Geometry: final body of the model. Coordinates: model frame, mm. Face numbers are marked on the shaded views. A direction names the side the tool comes from. Round coordinates to 2 decimals unless told otherwise and drop trailing zeros. Loops run counter-clockwise (first coordinate to the right, second up) from the corner with the lowest first, then second, coordinate; pieces in that order, holes last. Notation, with made-up numbers: (61, 22.25) - (111, 22.25) arc R32 ccw to (111, 50.25) - close; hole circle Ø3 at (19.25, -6). An arc over 180 degrees is marked (long way). Answer in a Markdown table with one row per item. Add a question column.
from build123d import *

# Parameters (mm, degrees)
SKETCH1_R           = 1.5
BOSS_EXTRUDE1_DEPTH = 1.6
SKETCH2_W           = 5
SKETCH2_H           = 25.4
BOSS_EXTRUDE2_DEPTH = 8


with BuildPart() as part:
    # Sketch1 → Boss-Extrude1 (new body)
    with BuildSketch(Plane(origin=(0, 0, 0), x_dir=(1, 0, 0), z_dir=(0, 1, 0))):
        with BuildLine():
            Line((1.5, 0), (98.5, 0))
            ThreePointArc((98.5, 0), (99.560660172, 0.439339828), (100, 1.5))
            Line((100, 1.5), (100, 78.5))
            ThreePointArc((100, 78.5), (99.560660172, 79.560660172), (98.5, 80))
            Line((98.5, 80), (1.5, 80))
            ThreePointArc((1.5, 80), (0.439339828, 79.560660172), (0, 78.5))
            Line((0, 78.5), (0, 1.5))
            ThreePointArc((0, 1.5), (0.439339828, 0.439339828), (1.5, 0))
        make_face()
        with Locations(Location((4, 4, 0), (0, 0, 270))):
            Circle(SKETCH1_R, mode=Mode.SUBTRACT)
        with Locations(Location((96, 76, 0), (0, 0, 270))):
            Circle(SKETCH1_R, mode=Mode.SUBTRACT)
        with Locations(Location((96, 4, 0), (0, 0, 270))):
            Circle(SKETCH1_R, mode=Mode.SUBTRACT)
        with Locations(Location((4, 76, 0), (0, 0, 270))):
            Circle(SKETCH1_R, mode=Mode.SUBTRACT)
    extrude(amount=BOSS_EXTRUDE1_DEPTH)

    # Sketch2 → Boss-Extrude2 (add)
    with BuildSketch(Plane(origin=(0, 1.6, 0), x_dir=(1, 0, 0), z_dir=(0, 1, 0))):
        with Locations((14.261833114, 15.332116758)):
            Rectangle(SKETCH2_W, SKETCH2_H)
        with Locations((13.597516255, 57.170048516)):
            Rectangle(SKETCH2_W, SKETCH2_H)
        with Locations((89.647028889, 60.563234223)):
            Rectangle(SKETCH2_W, SKETCH2_H)
        with Locations((86.389643886, 19.240978761)):
            Rectangle(SKETCH2_W, SKETCH2_H)
        with Locations((42.820913135, 59.911757222)):
            Rectangle(SKETCH2_W, SKETCH2_H)
        with Locations((68.613628586, 59.818689079)):
            Rectangle(SKETCH2_W, SKETCH2_H)
        with Locations((35.760574132, 15.239048615)):
            Rectangle(SKETCH2_W, SKETCH2_H)
        with Locations((64.518630297, 14.959844186)):
            Rectangle(SKETCH2_W, SKETCH2_H)
    extrude(amount=BOSS_EXTRUDE2_DEPTH)


solid = part.part
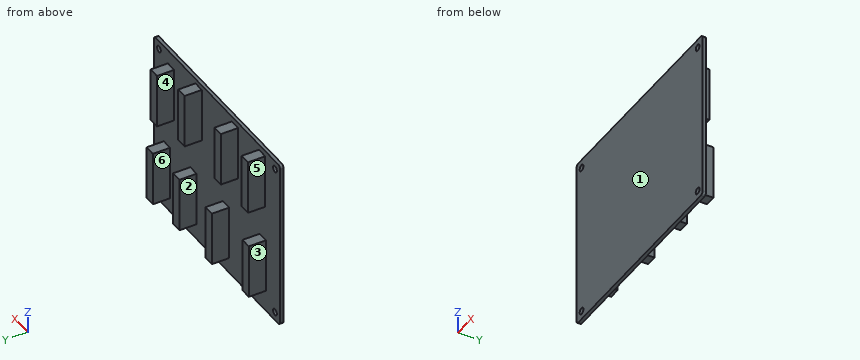
1) Material intervals for line 1 along X through (y, z) = (0.7, -4); line 2 along X through (y, z) = (5.25, -4); line 3 along Z through (x, y) = (96, 1.05), sorted ascending. Write a range as from..to.
2) Pull-direction query (X, two-part tool) for the marked faces 1, 2 and 3; classes: pulls with the +X half, pulls with the -X half, needs draft (parallel to the pull), parting line crosses it, or undercut.
3) Section D-D, the plane x = 14. Return the cut outline in (y, z).
4) Reachability of the marked faces 4, 5 and 6 from +Z, -Z, +X, -X, +Y, -Y: full face, straight path, thin tool, end or side. Return the list, or none.
5) Section A-A, the plane y = 6. Give the number of separate pieces and of enclosed holes in the cut face, and give its area (3 significant figures).
6) Section C-C, the plane x = 96. Return the cut outline in (y, z), and give its area (3 significant figures).
7) Contact query for flat-ended pins moving along their axis: pin 1 Ø1.5 at (x, y) = (36.5, 5.5) entering from -Z; pin 2 Ø1.8 at (x, z) = (96, -76) entering from +Y; pin 3 Ø1.5 at (y, z) = (7, -11) entering from -X; pin 4 Ø2.5 at (y, z) = (7, -64.5) entering from +X. Output: stop coordinate, or through.
8) Section B-B, the plane z = -4. Return the cut outline in (x, y), and give its area (3 significant figures).
Evaluation:
| question | item | result |
|---|---|---|
| 1 | line 1 | x = 0..2.5, 5.5..94.5, 97.5..100 |
| 1 | line 2 | x = 11.76..16.76, 33.26..38.26, 62.02..67.02 |
| 1 | line 3 | z = -80..-77.5, -74.5..-5.5, -2.5..0 |
| 2 | face 1 | needs draft |
| 2 | face 2 | undercut |
| 2 | face 3 | pulls with the -X half |
| 3 | outline | (0, -80) - (1.6, -80) - (1.6, -69.87) - (9.6, -69.87) - (9.6, -44.47) - (1.6, -44.47) - (1.6, -28.03) - (9.6, -28.03) - (9.6, -2.63) - (1.6, -2.63) - (1.6, 0) - (0, 0) - close |
| 4 | face 4 | +Z, -Z, +Y |
| 4 | face 5 | +Z, -X, +Y |
| 4 | face 6 | -Z, +Y |
| 5 | separate pieces | 8 |
| 5 | enclosed holes | 0 |
| 5 | area | 1,020 mm² |
| 6 | outline | (0, -80) - (1.6, -80) - (1.6, -77.5) - (0, -77.5) - close; (0, -74.5) - (1.6, -74.5) - (1.6, -5.5) - (0, -5.5) - close; (0, -2.5) - (1.6, -2.5) - (1.6, 0) - (0, 0) - close |
| 6 | area | 118 mm² |
| 7 | pin 1 | stops at z = -27.94 |
| 7 | pin 2 | passes through |
| 7 | pin 3 | stops at x = 11.76 |
| 7 | pin 4 | stops at x = 92.15 |
| 8 | outline | (0, 0) - (2.5, 0) - (2.5, 1.6) - (0, 1.6) - close; (5.5, 0) - (94.5, 0) - (94.5, 1.6) - (67.02, 1.6) - (67.02, 9.6) - (62.02, 9.6) - (62.02, 1.6) - (38.26, 1.6) - (38.26, 9.6) - (33.26, 9.6) - (33.26, 1.6) - (16.76, 1.6) - (16.76, 9.6) - (11.76, 9.6) - (11.76, 1.6) - (5.5, 1.6) - close; (97.5, 0) - (100, 0) - (100, 1.6) - (97.5, 1.6) - close |
| 8 | area | 270 mm² |
